Work out the finished part from the listing and answer in its coordinate system (mm). Round coordinates to 2 decimals unless told otherwise and drop trailing zeros. Order: outer loops, then holes, each group sorted by start corner. A loop starts at its lowest first (then second) coordinate and runs counter-clockwise, first axis right, second up. Notation, with made-up numbers: (30, 38) - (88, 38) arc R23 ccw to (88, 76) - close; hole circle Ø11 at (6.25, 21.25). An arc over 180 degrees is marked (long way). Put each result on its own line as item: value.
```python
from build123d import *

# Parameters (mm, degrees)
SKIZZE1_W                       = 410
SKIZZE1_H                       = 300
AUFSATZ_LINEAR_AUSTRAGEN1_DEPTH = 5
SKIZZE2_W                       = 46.676040128
SKIZZE2_H                       = 49.6
SCHNITT_LINEAR_AUSTRAGEN1_DEPTH = 5
LINEARES_MUSTER1_COUNT          = 4
LINEARES_MUSTER1_PITCH          = 99.9
SKIZZE3_W                       = 27.663601369
SKIZZE3_H                       = 49.6
SCHNITT_LINEAR_AUSTRAGEN2_DEPTH = 5
LINEARES_MUSTER2_COUNT          = 3
LINEARES_MUSTER2_PITCH          = 99.9
SKIZZE4_W                       = 49.6
SKIZZE4_H                       = 5
SCHNITT_LINEAR_AUSTRAGEN3_DEPTH = 5
LINEARES_MUSTER3_COUNT          = 3
LINEARES_MUSTER3_PITCH          = 99.9


with BuildPart() as part:
    # Skizze1 → Aufsatz-Linear austragen1 (new body)
    with BuildSketch(Plane.XY):
        with Locations((205, 150)):
            Rectangle(SKIZZE1_W, SKIZZE1_H)
    extrude(amount=AUFSATZ_LINEAR_AUSTRAGEN1_DEPTH)

    # Skizze2 → Schnitt-Linear austragen1 (cut)
    with BuildSketch(Plane.XY.offset(5)):
        with Locations((-18.338020064, 299.85)):
            Rectangle(SKIZZE2_W, SKIZZE2_H)
    schnitt_linear_austragen1 = extrude(amount=-SCHNITT_LINEAR_AUSTRAGEN1_DEPTH, mode=Mode.SUBTRACT)

    # Lineares Muster1: Schnitt-Linear austragen1 ×4
    with Locations(*[(0, -i * LINEARES_MUSTER1_PITCH, 0) for i in range(1, LINEARES_MUSTER1_COUNT)]):
        add(schnitt_linear_austragen1, mode=Mode.SUBTRACT)

    # Skizze3 → Schnitt-Linear austragen2 (cut)
    with BuildSketch(Plane.XY.offset(5)):
        with Locations((418.831800685, 249.9)):
            Rectangle(SKIZZE3_W, SKIZZE3_H)
    schnitt_linear_austragen2 = extrude(amount=-SCHNITT_LINEAR_AUSTRAGEN2_DEPTH, mode=Mode.SUBTRACT)

    # Lineares Muster2: Schnitt-Linear austragen2 ×3
    with Locations(*[(0, -i * LINEARES_MUSTER2_PITCH, 0) for i in range(1, LINEARES_MUSTER2_COUNT)]):
        add(schnitt_linear_austragen2, mode=Mode.SUBTRACT)

    # Skizze4 → Schnitt-Linear austragen3 (cut)
    with BuildSketch(Plane.XY.offset(5)):
        with Locations((104.75, 32.5)):
            Rectangle(SKIZZE4_W, SKIZZE4_H)
    schnitt_linear_austragen3 = extrude(amount=-SCHNITT_LINEAR_AUSTRAGEN3_DEPTH, mode=Mode.SUBTRACT)

    # Lineares Muster3: Schnitt-Linear austragen3 ×3
    with Locations(*[(i * LINEARES_MUSTER3_PITCH, 0, 0) for i in range(1, LINEARES_MUSTER3_COUNT)]):
        add(schnitt_linear_austragen3, mode=Mode.SUBTRACT)


solid = part.part
```
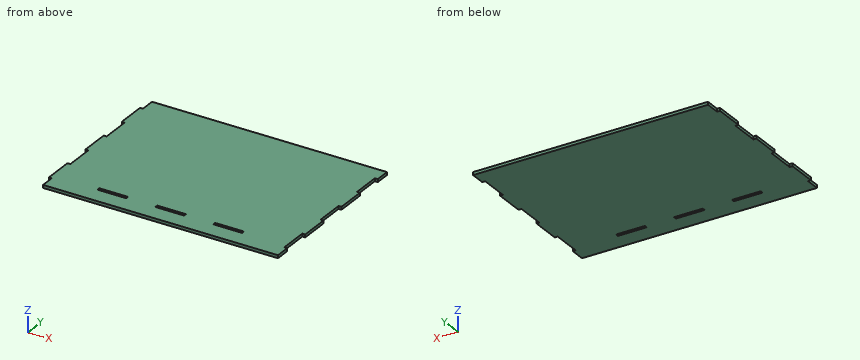
1) A cutting plane is placed at A-A on x = 194.5. Write down the section's boundary in (y, z), then the cut area to 4 significant figures.
Findings below:
outline: (0, 0) - (30, 0) - (30, 5) - (0, 5) - close; (35, 0) - (300, 0) - (300, 5) - (35, 5) - close
area: 1,475 mm2
2) Given pin 1 Ø2.5 at (x, z) = (2, 3.5) entering from +Y; pin 2 Ø1.5 at (y, z) = (284.5, 3) entering from -X, each flat-ended and moving along its own axis, determine where each tip first touches the part or whether it passes through.
Findings below:
pin 1: stops at y = 275.05
pin 2: stops at x = 5
3) Straight lines are drawn through the part: L1, parallel to Y at x = 196.5, z = 1.1; L2, parallel to X at y = 183, z = 1.15; L3, parallel to X at y = 62, z = 4.05. For each, find the intervals that lie inside material, in ascending order. Write a range as from..to.
Findings below:
L1: y = 0..30, 35..300
L2: x = 5..410
L3: x = 0..405
4) A cutting plane is placed at B-B on z = 3.45. Give the number of separate pieces and of enclosed holes in the cut face, then the cut area to 3 significant figures.
Findings below:
separate pieces: 1
enclosed holes: 3
area: 121,000 mm2
